Autodesk Inventor part; units mm, degrees
ref_plane "YZ Plane" through (0, 0, 0) normal (1, 0, 0) x (0, 1, 0)
ref_plane "XZ Plane" through (0, 0, 0) normal (0, 1, 0) x (-1, 0, 0)
ref_plane "XY Plane" through (0, 0, 0) normal (0, 0, 1) x (1, 0, 0)
sketch "Sketch1" plane through (0, 0, 0) normal (1, 0, 0) x (0, 1, 0)
  line L0 (0, 0) -> (300, 0)
  line L1 (300, 0) -> (300, 19.05)
  line L2 (300, 19.05) -> (0, 19.05)
  line L3 (0, 19.05) -> (0, 0)
  dimension "d0" = 300
  dimension "d1" = 19.05
extrude "Extrusion1" add sketch "Sketch1" along normal blind 6.35
sketch "Sketch2" plane through (6.35, 0, 0) normal (1, 0, 0) x (0, 0, -1)
  line L0 (0, 300) -> (-19.05, 300)
  line L1 (-19.05, 300) -> (-19.05, 0)
  line L2 (-19.05, 0) -> (0, 0)
  point P0 (-9.525, 285)
  point P1 (-9.525, 150)
  point P2 (-9.525, 15)
  dimension "d4" = 15
  dimension "d5" = 19.05
  dimension "d6" = 9.525
  dimension "d7" = 15
  dimension "d8" = 9.525
  dimension "d9" = 9.525
  dimension "d10" = 150
hole "Hole1" at (6.35, 285, 9.525) at (6.35, 150, 9.525) at (6.35, 15, 9.525) direction (-1, 0, 0) diameter 2.4638 end through all
sketch "Sketch5" plane through (6.35, 0, 0) normal (1, 0, 0) x (0, 0, -1)
  line L0 (-14.05, 270) -> (-5, 270)
  line L1 (-5, 270) -> (-5, 245)
  line L2 (-5, 245) -> (-14.05, 245)
  line L3 (-14.05, 245) -> (-14.05, 270)
  line L4 (-14.05, 205) -> (-5, 205)
  line L5 (-5, 205) -> (-5, 165)
  line L6 (-5, 165) -> (-14.05, 165)
  line L7 (-14.05, 165) -> (-14.05, 205)
  line L8 (-14.05, 135) -> (-5, 135)
  line L9 (-5, 135) -> (-5, 95)
  line L10 (-5, 95) -> (-14.05, 95)
  line L11 (-14.05, 95) -> (-14.05, 135)
  line L12 (-14.05, 55) -> (-5, 55)
  line L13 (-5, 55) -> (-5, 30)
  line L14 (-5, 30) -> (-14.05, 30)
  line L15 (-14.05, 30) -> (-14.05, 55)
  line L16 (0, 0) -> (0, 300)
  line L17 (-19.05, 300) -> (-19.05, 0)
  line L18 (0, 300) -> (-19.05, 300)
  line L19 (-19.05, 0) -> (0, 0)
  dimension "d44" = 5
  dimension "d45" = 5
  dimension "d46" = 30
  dimension "d47" = 30
  dimension "d48" = 55
  dimension "d49" = 95
  dimension "d50" = 135
  dimension "d51" = 55
  dimension "d52" = 95
  dimension "d53" = 135
extrude "Extrusion2" cut sketch "Sketch5" against normal through all contours L0 L1 L2 L3 | L4 L5 L6 L7 | L8 L9 L10 L11 | L12 L13 L14 L15
fillet "Fillet1" radius 3.175 1 edges at (3.175, 270, 5)
fillet "Fillet2" radius 3.175 1 edges at (3.175, 270, 14.05)
fillet "Fillet3" radius 3.175 1 edges at (3.175, 245, 5)
fillet "Fillet4" radius 3.175 1 edges at (3.175, 245, 14.05)
fillet "Fillet5" radius 3.175 1 edges at (3.175, 205, 5)
fillet "Fillet6" radius 3.175 1 edges at (3.175, 205, 14.05)
fillet "Fillet7" radius 3.175 1 edges at (3.175, 165, 5)
fillet "Fillet8" radius 3.175 1 edges at (3.175, 165, 14.05)
fillet "Fillet9" radius 3.175 1 edges at (3.175, 95, 5)
fillet "Fillet10" radius 3.175 1 edges at (3.175, 135, 5)
fillet "Fillet11" radius 3.175 1 edges at (3.175, 135, 14.05)
fillet "Fillet12" radius 3.175 1 edges at (3.175, 95, 14.05)
fillet "Fillet13" radius 3.175 1 edges at (3.175, 55, 5)
fillet "Fillet14" radius 3.175 1 edges at (3.175, 55, 14.05)
fillet "Fillet15" radius 3.175 1 edges at (3.175, 30, 14.05)
fillet "Fillet16" radius 3.175 1 edges at (3.175, 30, 5)
sketch "Sketch7" plane through (0, 0, 0) normal (0, 0, -1) x (-1, 0, 0)
  line L0 (0, 300) -> (-6.35, 300)
  line L1 (0, 0) -> (-6.35, 0)
  line L2 (-6.35, 0) -> (-6.35, 300)
  point P0 (-3.175, 7.5)
  point P1 (-3.175, 22.5)
  point P2 (-3.175, 142.5)
  point P3 (-3.175, 157.5)
  point P4 (-3.175, 277.5)
  point P5 (-3.175, 292.5)
  dimension "d72" = 7.5
  dimension "d73" = 22.5
  dimension "d74" = 142.5
  dimension "d78" = 7.5
  dimension "d79" = 22.5
  dimension "d82" = 142.5
  dimension "d83" = 6.35
  dimension "d84" = 3.175
  dimension "d85" = 3.175
  dimension "d88" = 3.175
  dimension "d89" = 3.175
  dimension "d92" = 3.175
  dimension "d93" = 3.175
hole "Hole3" at (3.175, 7.5, 0) at (3.175, 22.5, 0) at (3.175, 142.5, 0) at (3.175, 157.5, 0) at (3.175, 277.5, 0) at (3.175, 292.5, 0) direction (0, 0, 1) diameter 3.302 end through all
equation "\"d45\" = d44"
equation "\"d47\" = d46"
equation "\"d51\" = d48"
equation "\"d52\" = d49"
equation "\"d53\" = d50"
equation "\"d87\" = d84"
equation "\"d91\" = d89"
properties part number "slides"
Can you work these out from the model? Positions are in its coordinate system, mm. A direction names the side the tool comes from. Round coordinates to 2 decimals unless told otherwise and drop trailing zeros. Loops run counter-clockwise (first coordinate to the right, second up) from the corner with the lowest first, then second, coordinate; pieces in that order, holes last. Notation, with made-up numbers: (-18.5, -14) -> (4.5, -14) arc R13 cw to (4.5, 5) -> close; hole circle Ø4 at (87, -30.5). An arc over 180 degrees is marked (long way). One line per item, written item: value. Start each with the question number.
1. For faces 1 (the flat face through (0, 148, 10)), 2 (the flat face through (3, 185, 14.05)), which set-ups out of +Z, -Z, +X, -X, +Y, -Y let a thin tool reach every point of the face, with its end or its side?
2. If we mould it in two halves opening along Z, with no side actions, what happens to faces 3 (the flat face through (3, 185, 5)), 4 (the flat face through (3, 0, 10)), 5 (the flat face through (3, 152, 19.05))? For each: pulls with the +Z half, pulls with the -Z half, needs draft (parallel to the pull), parting line crosses it, or undercut.
3. If we section it at A-A, the plane y = 193.5: Write out the boundary of the cut face in (x, z), then the cut area to 3 significant figures.
4. If I drill on probe 1 along Y at (x, z) = (1, 8); probe 2 along Z at (x, y) = (4.5, 34.5); probe 3 along X at (y, z) = (292.5, 13.5), over which ranges is the centre line in solid material (lowest first)?
Calculated:
1. face 1: +Z, -Z, -X, +Y, -Y
1. face 2: +X, -X
2. face 3: undercut
2. face 4: needs draft
2. face 5: pulls with the +Z half
3. outline: (0, 0) -> (6.35, 0) -> (6.35, 5) -> (0, 5) -> close; (0, 14.05) -> (6.35, 14.05) -> (6.35, 19.05) -> (0, 19.05) -> close
3. area: 63.5 mm²
4. probe 1: y = 0 to 30, 55 to 95, 135 to 165, 205 to 245, 270 to 300
4. probe 2: z = 0 to 5, 14.05 to 19.05
4. probe 3: x = 0 to 1.52, 4.83 to 6.35
